Can you work these out from the model? Positions are in its coordinate system, mm. A direction names the side the tool comes from. Give positions to 0.01 mm unless a question says otherwise; leave off trailing zeros. Loops run counter-clockwise (first coordinate to the right, second up) from the corner with the lowest first, then second, coordinate; pieces in that order, holes last. Notation, with made-up numbers: (-19, -33.75) -> (8, -33.75) arc R27 cw to (8, -13.75) -> close; hole circle Ø10 at (-32, 78.5). An arc over 180 degrees is marked (long way). One line per question, with ' | ' between items.
from build123d import *

# Parameters (mm, degrees)
BOSS_EXTRUDE1_DEPTH      = 1.6002
CUT_EXTRUDE1_DEPTH       = 2.6002
CUT_EXTRUDE2_DEPTH       = 2.6002
CUT_EXTRUDE3_DEPTH       = 2.6002
CUT_EXTRUDE4_DEPTH       = 2.6002
SKETCH6_W                = 135.636
SKETCH6_H                = 61.722
BOSS_EXTRUDE2_DEPTH      = 11
SKETCH7_W                = 135.128
SKETCH7_H                = 61.214
CUT_EXTRUDE5_DEPTH       = 11
SKETCH8_W                = 75.184
SKETCH8_H                = 24.384
CUT_EXTRUDE6_DEPTH       = 2.6002
SKETCH9_W                = 11.792676588
SKETCH9_H                = 1.790289347
CUT_EXTRUDE7_DEPTH       = 13.6002
M2_CLEARANCE_HOLE1_D     = 2.39776
M2_CLEARANCE_HOLE1_DEPTH = 1.6002
M4_CLEARANCE_HOLE2_D     = 4.68589235
M4_CLEARANCE_HOLE2_DEPTH = 1.6002


with BuildPart() as part:
    # Sketch1 → Boss-Extrude1 (new body)
    with BuildSketch(Plane.XY.offset(1.6002)):
        Polygon((6.35, 70.612), (0, 64.262), (0, 3.81), (6.35, -2.54), (147.066, -2.54), (153.416, 3.81), (153.416, 64.262), (147.066, 70.612), align=None)
    extrude(amount=-BOSS_EXTRUDE1_DEPTH)

    # Sketch2 → Cut-Extrude1 (cut, through all)
    with BuildSketch(Plane(origin=(0, 0, 0), x_dir=(-1, 0, 0), z_dir=(0, 0, -1))):
        with BuildLine():
            Line((-153.416, 9.525), (-153.416, 5.715))
            Line((-153.416, 5.715), (-149.606, 5.715))
            ThreePointArc((-149.606, 5.715), (-147.701, 7.62), (-149.606, 9.525))
            Line((-149.606, 9.525), (-153.416, 9.525))
        make_face()
    extrude(amount=-CUT_EXTRUDE1_DEPTH, mode=Mode.SUBTRACT)

    # Sketch3 → Cut-Extrude2 (cut, through all)
    with BuildSketch(Plane(origin=(0, 0, 0), x_dir=(-1, 0, 0), z_dir=(0, 0, -1))):
        with BuildLine():
            Line((-153.416, 62.357), (-153.416, 58.547))
            Line((-153.416, 58.547), (-149.606, 58.547))
            ThreePointArc((-149.606, 58.547), (-147.701, 60.452), (-149.606, 62.357))
            Line((-149.606, 62.357), (-153.416, 62.357))
        make_face()
    extrude(amount=-CUT_EXTRUDE2_DEPTH, mode=Mode.SUBTRACT)

    # Sketch4 → Cut-Extrude3 (cut, through all)
    with BuildSketch(Plane(origin=(0, 0, 0), x_dir=(-1, 0, 0), z_dir=(0, 0, -1))):
        with BuildLine():
            Line((0, 58.547), (0, 62.357))
            Line((0, 62.357), (-3.81, 62.357))
            ThreePointArc((-3.81, 62.357), (-5.715, 60.452), (-3.81, 58.547))
            Line((-3.81, 58.547), (0, 58.547))
        make_face()
    extrude(amount=-CUT_EXTRUDE3_DEPTH, mode=Mode.SUBTRACT)

    # Sketch5 → Cut-Extrude4 (cut, through all)
    with BuildSketch(Plane(origin=(0, 0, 0), x_dir=(-1, 0, 0), z_dir=(0, 0, -1))):
        with BuildLine():
            Line((0, 5.715), (0, 9.525))
            Line((0, 9.525), (-3.81, 9.525))
            ThreePointArc((-3.81, 9.525), (-5.715, 7.62), (-3.81, 5.715))
            Line((-3.81, 5.715), (0, 5.715))
        make_face()
    extrude(amount=-CUT_EXTRUDE4_DEPTH, mode=Mode.SUBTRACT)

    # Sketch6 → Boss-Extrude2 (add)
    with BuildSketch(Plane.XY.offset(1.6002)):
        with Locations((74.93, 33.909)):
            Rectangle(SKETCH6_W, SKETCH6_H)
    extrude(amount=BOSS_EXTRUDE2_DEPTH)

    # Sketch7 → Cut-Extrude5 (cut)
    with BuildSketch(Plane.XY.offset(12.6002)):
        with Locations((74.93, 33.909)):
            Rectangle(SKETCH7_W, SKETCH7_H)
    extrude(amount=-CUT_EXTRUDE5_DEPTH, mode=Mode.SUBTRACT)

    # Sketch8 → Cut-Extrude6 (cut, through all)
    with BuildSketch(Plane.XY.offset(1.6002)):
        with Locations((92.71, 34.036)):
            Rectangle(SKETCH8_W, SKETCH8_H)
    extrude(amount=-CUT_EXTRUDE6_DEPTH, mode=Mode.SUBTRACT)

    # Sketch9 → Cut-Extrude7 (cut, through all)
    with BuildSketch(Plane(origin=(0, 0, 0), x_dir=(-1, 0, 0), z_dir=(0, 0, -1))):
        with Locations((-17.905053156, 12.47860787)):
            Rectangle(SKETCH9_W, SKETCH9_H)
    extrude(amount=-CUT_EXTRUDE7_DEPTH, mode=Mode.SUBTRACT)

    # M2 Clearance Hole1
    with Locations(Plane.XY.offset(1.6002)):
        with Locations((127.4445, 6.98246), (127.44958, 11.303), (57.4548, 7.03326), (57.43956, 11.32332)):
            Hole(M2_CLEARANCE_HOLE1_D / 2, depth=M2_CLEARANCE_HOLE1_DEPTH)

    # M4 Clearance Hole2
    with Locations(Plane.XY.offset(1.6002)):
        with Locations((34.22065157, 13.205568935)):
            Hole(M4_CLEARANCE_HOLE2_D / 2, depth=M4_CLEARANCE_HOLE2_DEPTH)


solid = part.part
Q1. On a 3-axis mill with a long thin cutter (end or side, diameter ignored), from which of +Z, -Z, +X, -X, +Y, -Y can I reach the whole of each face in a straight line? I mean faces 4 (the face through (74, 64.77, 7)), 5 (the face through (74, 3.302, 7)), 6 (the face through (7.112, 33, 7)). Say none if no direction works.
Entries:
face 4: +Z, +X, -X, +Y | face 5: +Z | face 6: +Z, -X, +Y, -Y
Q2. If we section it at B-B (y = 23.5): Write out the boundary of the cut face in (x, z).
Entries:
outline: (0, 0) -> (55.12, 0) -> (55.12, 1.6) -> (7.37, 1.6) -> (7.37, 12.6) -> (7.11, 12.6) -> (7.11, 1.6) -> (0, 1.6) -> close; (130.3, 0) -> (153.42, 0) -> (153.42, 1.6) -> (142.75, 1.6) -> (142.75, 12.6) -> (142.49, 12.6) -> (142.49, 1.6) -> (130.3, 1.6) -> close
Q3. If we section it at C-C (z = 5.25): Write out the boundary of the cut face in (x, y).
Entries:
outline: (7.11, 3.05) -> (142.75, 3.05) -> (142.75, 64.77) -> (7.11, 64.77) -> close; hole (7.37, 3.3) -> (142.49, 3.3) -> (142.49, 64.52) -> (7.37, 64.52) -> close
Q4. If we mould it in two halves opening along Y, with no side actions, what happens to faces 1 (the face through (142.494, 33, 7)), 2 (the face through (3.13, 0.68, 0.81)), 3 (the face through (142.748, 33, 7))? For each: pulls with the +Y half, pulls with the -Y half, needs draft (parallel to the pull), parting line crosses it, or undercut.
Entries:
face 1: undercut | face 2: pulls with the -Y half | face 3: needs draft
Q5. If we section it at A-A (x = 95.5): Write out the boundary of the cut face in (y, z).
Entries:
outline: (-2.54, 0) -> (21.84, 0) -> (21.84, 1.6) -> (3.3, 1.6) -> (3.3, 12.6) -> (3.05, 12.6) -> (3.05, 1.6) -> (-2.54, 1.6) -> close; (46.23, 0) -> (70.61, 0) -> (70.61, 1.6) -> (64.77, 1.6) -> (64.77, 12.6) -> (64.52, 12.6) -> (64.52, 1.6) -> (46.23, 1.6) -> close
Q6. If we section it at D-D (x = 39): Write out the boundary of the cut face in (y, z), plus the area to 3 significant figures.
Entries:
outline: (-2.54, 0) -> (70.61, 0) -> (70.61, 1.6) -> (64.77, 1.6) -> (64.77, 12.6) -> (64.52, 12.6) -> (64.52, 1.6) -> (3.3, 1.6) -> (3.3, 12.6) -> (3.05, 12.6) -> (3.05, 1.6) -> (-2.54, 1.6) -> close | area: 123 mm²
Q7. For pin 1 Ø5 at (x, y) = (17, 25) entering from +Z; pin 2 Ø1.3 at (x, z) = (1, 1) entering from +Y; pin 3 Ø0.8 at (x, z) = (1, 1) entering from +Y, each with a flat end and sliding along its axis, tell me the tip position at first contact or that it passes through.
Entries:
pin 1: z = 1.6 | pin 2: y = 65.91 | pin 3: y = 65.66
Q8. If I drill on probe 1 along X at (y, z) = (59.5, 6.25); probe 2 along Y at (x, z) = (127, 10.25); probe 3 along Y at (x, z) = (77.5, 1.5), over which ranges is the centre line in solid material (lowest first)? Write a range as from..to.
Entries:
probe 1: 7.11..7.37, 142.49..142.75 | probe 2: 3.05..3.3, 64.52..64.77 | probe 3: -2.54..21.84, 46.23..70.61
